Geometry check sheet. Reference: the model listing, model coordinates, mm. Face numbers are marked on the shaded views. Coordinates: 2 decimals unless noted, no trailing zeros. Loops run counter-clockwise (first coordinate to the right, second up) from the corner with the lowest first, then second, coordinate; pieces in that order, holes last.
Autodesk Inventor part; units mm, degrees
ref_plane "YZ Plane" through (0, 0, 0) normal (1, 0, 0) x (0, 1, 0)
ref_plane "XZ Plane" through (0, 0, 0) normal (0, 1, 0) x (-1, 0, 0)
ref_plane "XY Plane" through (0, 0, 0) normal (0, 0, 1) x (1, 0, 0)
sketch "Sketch1" plane through (0, 0, 0) normal (0, 1, 0) x (-1, 0, 0)
  line L0 (0, 0) -> (34, 0)
  line L1 (34, 0) -> (34, -52.1)
  line L2 (34, -52.1) -> (0, -52.1)
  line L3 (0, -52.1) -> (0, 0)
  circle A0 centre (28, -4.85) radius 1.6
  line L4 (28, -8.0832) -> (25.2, -6.4666)
  line L5 (25.2, -6.4666) -> (25.2, -3.2334)
  line L6 (25.2, -3.2334) -> (28, -1.6168)
  line L7 (28, -1.6168) -> (30.8, -3.2334)
  line L8 (30.8, -3.2334) -> (30.8, -6.4666)
  line L9 (30.8, -6.4666) -> (28, -8.0832)
  line L10 (17, 0) -> (17, -52.1) construction
  line L11 (0, -26.05) -> (34, -26.05) construction
  line L12 (17, -19.8) -> (14, -19.8)
  line L13 (14, -19.8) -> (14, -32.3)
  line L14 (14, -32.3) -> (17, -32.3)
  line L15 (17, -32.3) -> (17, -19.8)
  line L16 (23.2, -19.8) -> (20.2, -19.8)
  line L17 (20.2, -19.8) -> (20.2, -32.3)
  line L18 (20.2, -32.3) -> (23.2, -32.3)
  line L19 (23.2, -32.3) -> (23.2, -19.8)
  dimension "d0" = 34
  dimension "d1" = 52.1
  dimension "d2" = 3.2
  dimension "d3" = 4.85
  dimension "d4" = 6
  dimension "d5" = 5.6
  dimension "d18" = 3
  dimension "d19" = 12.5
  dimension "d20" = 3
  dimension "d21" = 12.5
  dimension "d22" = 19.8
  dimension "d23" = 3.2
extrude "Extrusion1" add sketch "Sketch1" along normal blind 4 contours L0 L1 L2 L3 | A0 | L4 L5 L6 L7 L8 L9 | L15 L14 L13 L12 | L19 L18 L17 L16
extrude "Extrusion2" cut sketch "Sketch1" along normal blind 2 contours L4 L5 L6 L7 L8 L9
extrude "Extrusion3" cut sketch "Sketch1" along normal blind 4 contours A0
pattern_linear "Rectangular Pattern1" count 2 spacing 42.4 along (0, 0, -1) count 2 spacing 22 along (1, 0, 0) of "Extrusion3", "Extrusion2"
extrude "Extrusion4" add sketch "Sketch1" against normal blind 15 contours L15 L14 L13 L12 | L19 L18 L17 L16
sketch "Sketch2" plane through (-14, -15, -19.8) normal (1, 0, 0) x (0, 0, -1)
  line L0 (0, 15) -> (12.5, 15)
  line L1 (0, 15) -> (0, 0)
  line L2 (12.5, 0) -> (0, 0)
  line L3 (12.5, 15) -> (12.5, 0)
  circle A0 centre (6.25, 6.25) radius 1.65
  point P0 (-19.8, 15)
  dimension "d26" = 3.3
  dimension "d27" = 12.5
  dimension "d28" = 6.25
  dimension "d29" = 6.25
extrude "Extrusion5" cut sketch "Sketch2" against normal up to surface (9.2 mm away) contours A0
fillet "Fillet1" radius 6.25 4 edges at (-15.5, -15, -19.8) (-15.5, -15, -32.3) (-21.7, -15, -19.8) (-21.7, -15, -32.3)
fillet "Fillet2" radius 4 4 edges at (-15.5, 0, -19.8) (-15.5, 0, -32.3) (-21.7, 0, -19.8) (-21.7, 0, -32.3)
fillet "Fillet3" radius 2 4 edges at (-34, 2, 0) (-34, 2, -52.1) (0, 2, 0) (0, 2, -52.1)
equation "\"d22\" = -0.5 * d19 + 0.5 * d1"
equation "\"d28\" = 0.5 * d27"
equation "\"d29\" = d28"
properties part number "encaixeDuplo"
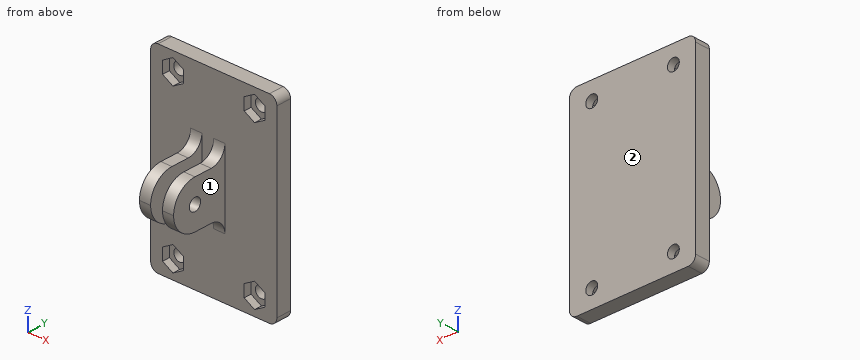
(1) Scan lines: L1, parallel to Z at x = -28, y = 2.75; L2, parallel to Y at x = -14.75, z = -26.05; L3, parallel to Y at x = -9, z = -36. Record each from-to range of solid material in increasing order.
Findings:
L1: z = -52.1 to -48.85, -45.65 to -6.45, -3.25 to 0
L2: y = -15 to -10.4, -7.1 to 4
L3: y = 0 to 4
(2) Draft check along X on the marked faces 1 and 2. Enter one of: +X half, -X half, draft (parallel to the pull), parting line (faces both ways), or undercut.
Findings:
face 1: +X half
face 2: draft
(3) Sectioned sample at B-B on z = -47.25. Record the cut outline in (x, y), and give its area (3 significant figures).
Findings:
outline: (-34, 0) - (-30.8, 0) - (-30.8, 2) - (-29.6, 2) - (-29.6, 4) - (-34, 4) - close; (-26.4, 2) - (-25.2, 2) - (-25.2, 0) - (-8.8, 0) - (-8.8, 2) - (-7.6, 2) - (-7.6, 4) - (-26.4, 4) - close; (-4.4, 2) - (-3.2, 2) - (-3.2, 0) - (0, 0) - (0, 4) - (-4.4, 4) - close
area: 101 mm2
(4) Gauge pin test, flat ends, axial feed: pin 1 Ø3 at (y, z) = (-11.5, -28.5) entering from -X; pin 2 Ø3.5 at (x, y) = (-15, -5) entering from -Z; pin 3 Ø6 at (y, z) = (-4, -20) entering from +X. Record the tip position at first contact, or that the pin passes through.
Findings:
pin 1: stops at x = -23.2
pin 2: stops at z = -32.37
pin 3: stops at x = -14
(5) Sectioned sample at D-D on z = -7. Record the cut outline in (x, y), and give its area (3 significant figures).
Findings:
outline: (-34, 0) - (-29.88, 0) - (-29.88, 2) - (-26.12, 2) - (-26.12, 0) - (-7.88, 0) - (-7.88, 2) - (-4.12, 2) - (-4.12, 0) - (0, 0) - (0, 4) - (-34, 4) - close
area: 121 mm2
(6) Sectioned sample at C-C on y = -12.25. Record the cut outline in (x, z), and give its area (3 significant figures).
Findings:
outline: (-23.2, -31.23) - (-20.2, -31.23) - (-20.2, -20.87) - (-23.2, -20.87) - close; (-17, -31.23) - (-14, -31.23) - (-14, -20.87) - (-17, -20.87) - close
area: 62.1 mm2
